from build123d import *

# Parameters (mm, degrees)
BOSS_EXTRUDE1_DEPTH     = 10
CUT_EXTRUDE2_DEPTH      = 14.114877049
SKETCH6_W               = 3.9
SKETCH6_H               = 6
BOSS_EXTRUDE3_DEPTH     = 4
SKETCH7_W               = 3.9
SKETCH7_H               = 3
REVOLVE1_ANGLE          = 180
SKETCH9_R               = 1.45
CUT_EXTRUDE3_DEPTH      = 5
SKETCH10_W              = 3.9
SKETCH10_H              = 6
BOSS_EXTRUDE4_DEPTH     = 4
REVOLVE2_ANGLE          = 180
SKETCH14_R              = 1.45
CUT_EXTRUDE4_DEPTH      = 5
BOSS_EXTRUDE7_DEPTH     = 3.7
BOSS_EXTRUDE17_DEPTH    = 3.75
CUT_EXTRUDE6_DEPTH      = 20
CUT_EXTRUDE6_DEPTH_BACK = 20
CUT_EXTRUDE7_DEPTH      = 20.702855123
CUT_EXTRUDE7_DEPTH_BACK = 20.702855123
CUT_EXTRUDE8_DEPTH      = 22.656407828
CUT_EXTRUDE8_DEPTH_BACK = 22.656407828


with BuildPart() as part:
    # Sketch2 → Boss-Extrude1 (new, symmetric)
    with BuildSketch(Plane(origin=(0, 0, 0), x_dir=(1, 0, 0), z_dir=(0, 1, 0))):
        Polygon((-3, 6), (3, 6), (6, 3), (6, -3), (3, -6), (-3, -6), (-6, -3), (-6, 3), align=None)
    extrude(amount=BOSS_EXTRUDE1_DEPTH, both=True)

    # Sketch5 → Cut-Extrude2 (cut, symmetric)
    with BuildSketch(Plane(origin=(0, 0, 0), x_dir=(0, 0, -1), z_dir=(1, 0, 0))):
        Polygon((0, 10), (6, 6.535898385), (6, 10), align=None)
    cut_extrude2 = extrude(amount=CUT_EXTRUDE2_DEPTH, both=True, mode=Mode.SUBTRACT)

    # Mirror3: Cut-Extrude2 across plane
    add(cut_extrude2.mirror(Plane.ZX), mode=Mode.SUBTRACT)

    # Sketch6 → Boss-Extrude3 (add, symmetric)
    with BuildSketch(Plane.XZ.offset(10)):
        with Locations((-4.05, 0)):
            Rectangle(SKETCH6_W, SKETCH6_H)
    boss_extrude3 = extrude(amount=BOSS_EXTRUDE3_DEPTH, both=True)

    # Sketch7 → Revolve1 (revolve)
    with BuildSketch(Plane.XZ.offset(14)):
        with Locations((-4.05, 1.5)):
            Rectangle(SKETCH7_W, SKETCH7_H)
    revolve1 = revolve(axis=Axis((-6, -14, 0), (1, 0, 0)), revolution_arc=REVOLVE1_ANGLE)

    # Sketch9 → Cut-Extrude3 (cut, symmetric)
    with BuildSketch(Plane.ZY.offset(6)):
        with Locations((0, -14)):
            Circle(SKETCH9_R)
    cut_extrude3 = extrude(amount=CUT_EXTRUDE3_DEPTH, both=True, mode=Mode.SUBTRACT)

    # Mirror5: Boss-Extrude3, Revolve1, Cut-Extrude3 across plane
    add(boss_extrude3.mirror(Plane(origin=(0, 0, 0), x_dir=(0, 0, 1), z_dir=(1, 0, 0))))
    add(revolve1.mirror(Plane(origin=(0, 0, 0), x_dir=(0, 0, 1), z_dir=(1, 0, 0))))
    add(cut_extrude3.mirror(Plane(origin=(0, 0, 0), x_dir=(0, 0, 1), z_dir=(1, 0, 0))), mode=Mode.SUBTRACT)

    # Sketch10 → Boss-Extrude4 (add, symmetric)
    with BuildSketch(Plane(origin=(0, 10, 0), x_dir=(1, 0, 0), z_dir=(0, 1, 0))):
        Rectangle(SKETCH10_W, SKETCH10_H)
    extrude(amount=BOSS_EXTRUDE4_DEPTH, both=True)

    # Sketch12 → Revolve2 (revolve)
    with BuildSketch(Plane(origin=(0, 14, 0), x_dir=(1, 0, 0), z_dir=(0, 1, 0))):
        Polygon((-1.95, 3), (-1.95, 0), (1.95, 0.003655936), (1.95, 3), align=None)
    revolve(axis=Axis((-1.95, 14, 0), (0.9999995606226393, 0, -0.0009374190783233235)), revolution_arc=REVOLVE2_ANGLE)

    # Sketch14 → Cut-Extrude4 (cut, symmetric)
    with BuildSketch(Plane.ZY.offset(1.95)):
        with Locations((0, 14)):
            Circle(SKETCH14_R)
    extrude(amount=CUT_EXTRUDE4_DEPTH, both=True, mode=Mode.SUBTRACT)

    # Sketch17 → Boss-Extrude7 (add)
    with BuildSketch(Plane(origin=(0, 10, 0), x_dir=(1, 0, 0), z_dir=(0, 1, 0))):
        Polygon((-6, -3), (-1.95, -3), (1.95, -3), (6, -3), (3, -6), (-3, -6), align=None)
    extrude(amount=BOSS_EXTRUDE7_DEPTH)

    # Sketch19 → Boss-Extrude17 (add)
    with BuildSketch(Plane.XZ.offset(10)):
        Polygon((-6, 3), (-2.1, 3), (2.1, 3), (6, 3), (3, 6), (-3, 6), align=None)
    extrude(amount=BOSS_EXTRUDE17_DEPTH)

    # Sketch15 → Cut-Extrude6 (cut, two sides: drawn at the far end of the back side and taken through both)
    with BuildSketch(Plane(origin=(0, 0, 0), x_dir=(1, 0, 0), z_dir=(0, 1, 0)).offset(-CUT_EXTRUDE6_DEPTH_BACK)):
        Polygon((0, 5.5), (-1, 4.5), (-1, 3.5), (1, 3.5), (1, 4.5), align=None)
        Polygon((1, -4.5), (0, -3.5), (-1, -4.5), (-1, -5.5), (1, -5.5), align=None)
    extrude(amount=CUT_EXTRUDE6_DEPTH + CUT_EXTRUDE6_DEPTH_BACK, mode=Mode.SUBTRACT)

    # Sketch20 → Cut-Extrude7 (cut, two sides: drawn at the far end of the back side and taken through both)
    with BuildSketch(Plane.ZY.offset(1.95).offset(-CUT_EXTRUDE7_DEPTH_BACK)):
        Polygon((3, 14), (8.338e-05, 16.999998681), (8.6017e-05, 17.537492691), (3, 17.537492691), (3.371623525, 17.537492691), (3.371623525, 14), align=None)
    extrude(amount=CUT_EXTRUDE7_DEPTH + CUT_EXTRUDE7_DEPTH_BACK, mode=Mode.SUBTRACT)

    # Sketch21 → Cut-Extrude8 (cut, two sides: drawn at the far end of the back side and taken through both)
    with BuildSketch(Plane(origin=(6, 0, 0), x_dir=(0, 0, -1), z_dir=(1, 0, 0)).offset(-CUT_EXTRUDE8_DEPTH_BACK)):
        Polygon((-3, -14), (0, -17), (0, -17.720731205), (-3.510483934, -17.720731205), (-3.510483934, -14.510483934), (-3.510483934, -14), align=None)
    extrude(amount=CUT_EXTRUDE8_DEPTH + CUT_EXTRUDE8_DEPTH_BACK, mode=Mode.SUBTRACT)


solid = part.part
Build history of the part. All positions in model axes, mm. A direction names the side the tool comes from. Give positions to 0.01 mm unless a question says otherwise; leave off trailing zeros. Order: outer loops, then holes, each group sorted by start corner. A loop starts at its lowest first (then second) coordinate and runs counter-clockwise, first axis right, second up. Notation, with made-up numbers: M -17.5,-8.5 L 17.5,-8.5 A4 cw 17.5,-3.5 Z; hole C 17.5,-19 d4. An arc over 180 degrees is marked long. Put each result on its own line as item: value.
Item 1: Slice it at A-A, the plane x = -4.5. Write the cut outline in (y, z).
From the geometry:
outline: M -17,0 A3 ccw -14,-3 L -8.27,-3 L -7.4,-4.5 L 7.4,-4.5 L 10,0 L 10,3 L 13.7,3 L 13.7,4.5 L -13.75,4.5 L -13.75,3 L -14,3 Z; hole C -14,0 d2.9
Item 2: Probe line 1 (Y direction, x = 3.8, z = 0); line 2 (Z direction, x = 3.2, y = -14); line 3 (X direction, y = -11, z = -1.5). List the from-to ranges inside material, lowest first. Write a range as [from, to].
From the geometry:
line 1: y = [-17, -15.45], [-12.55, 10]
line 2: z = [-3, -1.45], [1.45, 3]
line 3: x = [-6, -2.1], [2.1, 6]
Item 3: Slice it at D-D, the plane z = -1. Give the number of separate pieces and of enclosed holes in the cut face, plus the area to 3 significant figures.
From the geometry:
separate pieces: 4
enclosed holes: 0
area: 288 mm2
Item 4: Two-plate mould, pull along Y, no slides. Class faces 1 (the flat face through (4, 10, 1)), 2 (the cylindrical face through (4.077, -12.562, -0.189)), 3 (the flat face through (-4, 0, 5)): +Y half, -Y half, draft (parallel to the pull), parting line (faces both ways), or undercut.
From the geometry:
face 1: +Y half
face 2: undercut
face 3: draft
Item 5: Flat gauge pins, fed straight in: pin 1 Ø0.5 at (y, z) = (-2, -4) entering from -X; pin 2 Ø2 at (x, z) = (-0.5, -3) entering from -Y; pin 3 Ø2.5 at (x, z) = (0.5, 4) entering from -Y; pin 4 Ø2.5 at (y, z) = (14, 0) entering from +X. Where does each tip first touch, or does it go through?
From the geometry:
pin 1: stops at x = -5.25
pin 2: stops at y = -8.85
pin 3: stops at y = -13.75
pin 4: passes through
Item 6: 3-axis set-ups, long thin cutter, end or side, ignore diameter. For faces 4 (the flat face through (-1, 0, 5)), 5 (the flat face through (0, 11, -3)): which of +Z, -Z, +X, -X, +Y, -Y reach the whole face in a straight line?
From the geometry:
face 4: +Y, -Y
face 5: -Z, +X, -X, +Y
Item 7: Slice it at B-B, the plane y = 0.5. Write the cut outline in (x, z).
From the geometry:
outline: M -6,-3 L -3,-6 L 3,-6 L 6,-3 L 6,3 L 3,6 L -3,6 L -6,3 Z; hole M -1,-4.5 L 0,-5.5 L 1,-4.5 L 1,-3.5 L -1,-3.5 Z; hole M -1,4.5 L 0,3.5 L 1,4.5 L 1,5.5 L -1,5.5 Z
Item 8: Slice it at C-C, the plane y = -11.5. Write the cut outline in (x, z), plus the area to 3 significant figures.
From the geometry:
outline: M -6,-3 L -2.1,-3 L -2.1,3 L 2.1,3 L 2.1,-3 L 6,-3 L 6,3 L 3,6 L -3,6 L -6,3 Z; hole M -1,4.5 L 0,3.5 L 1,4.5 L 1,5.5 L -1,5.5 Z
area: 70.8 mm2
